Input: part model. Units: mm. Frame: model coordinates. Coordinates: 2 decimals unless noted, no trailing zeros. Write each loop counter-clockwise with the first axis right and the second up, starting at its lowest first coordinate (ties: lowest second). Pieces come first, ordered by that corner, then holes. Notation, with made-up numbers: (19.25, 47.5) - (50.25, 47.5) arc R11 cw to (50.25, 56.5) - close; hole circle Ø11 at (20, 75.25). An arc over 180 degrees is marked (long way). Put each result on its own line as item: value. Start each with the question number.
1. Cut plane B-B, the plane x = 85. Return loops of the section in (y, z).
2. Cut plane D-D, the plane y = 34. Return loops of the section in (x, z), and give its area (3 significant figures).
3. Cut plane C-C, the plane z = 1.15. Return loops of the section in (x, y), and give its area (3 significant figures).
4. Line query: line 1 (Y direction, x = 15, z = 1.2); line 2 (X direction, y = 5.5, z = 1.2); line 3 (X direction, y = 25.5, z = 0.5). Output: solid intervals per line, ascending.
5. Pull-direction query (Y, two-part tool) for faces 1 (the flat face through (49, 26, 0)), 2 (the cylindrical face through (13.4, 46.07, 0.79)); classes: released by +Y, released by -Y, zero draft, split by the parting line, or undercut.
6. Cut plane A-A, the plane y = 46. Return loops of the section in (x, z).
from build123d import *

# Parameters (mm, degrees)
ESQUISSE1_W             = 100
ESQUISSE1_H             = 52
ESQUISSE1_R             = 1.6
BOSS_EXTRU_1_DEPTH      = 1.6
ESQUISSE2_R             = 10
ENL_V_MAT_EXTRU_1_DEPTH = 113.723378232


with BuildPart() as part:
    # Esquisse1 → Boss.-Extru.1 (new body)
    with BuildSketch(Plane.XY):
        with Locations((50, 26)):
            Rectangle(ESQUISSE1_W, ESQUISSE1_H)
        with Locations((15, 46)):
            Circle(ESQUISSE1_R, mode=Mode.SUBTRACT)
        with Locations((85, 46)):
            Circle(ESQUISSE1_R, mode=Mode.SUBTRACT)
        with Locations((15, 6)):
            Circle(ESQUISSE1_R, mode=Mode.SUBTRACT)
        with Locations((85, 6)):
            Circle(ESQUISSE1_R, mode=Mode.SUBTRACT)
    extrude(amount=BOSS_EXTRU_1_DEPTH)

    # Esquisse2 → Enlèv. mat.-Extru.1 (cut, through all)
    with BuildSketch(Plane(origin=(0, 0, 0), x_dir=(-1, 0, 0), z_dir=(0, 0, -1))):
        with Locations((-100, 26)):
            Circle(ESQUISSE2_R)
        with Locations((0, 26)):
            Circle(ESQUISSE2_R)
    extrude(amount=-ENL_V_MAT_EXTRU_1_DEPTH, mode=Mode.SUBTRACT)


solid = part.part
Report:
1. outline: (0, 0) - (4.4, 0) - (4.4, 1.6) - (0, 1.6) - close; (7.6, 0) - (44.4, 0) - (44.4, 1.6) - (7.6, 1.6) - close; (47.6, 0) - (52, 0) - (52, 1.6) - (47.6, 1.6) - close
2. outline: (6, 0) - (94, 0) - (94, 1.6) - (6, 1.6) - close
2. area: 141 mm^2
3. outline: (0, 0) - (100, 0) - (100, 16) arc R10 cw to (100, 36) - (100, 52) - (0, 52) - (0, 36) arc R10 cw to (0, 16) - close; hole circle Ø3.2 at (15, 6); hole circle Ø3.2 at (15, 46); hole circle Ø3.2 at (85, 6); hole circle Ø3.2 at (85, 46)
3. area: 4,850 mm^2
4. line 1: y = 0 to 4.4, 7.6 to 44.4, 47.6 to 52
4. line 2: x = 0 to 13.48, 16.52 to 83.48, 86.52 to 100
4. line 3: x = 9.99 to 90.01
5. face 1: zero draft
5. face 2: undercut
6. outline: (0, 0) - (13.4, 0) - (13.4, 1.6) - (0, 1.6) - close; (16.6, 0) - (83.4, 0) - (83.4, 1.6) - (16.6, 1.6) - close; (86.6, 0) - (100, 0) - (100, 1.6) - (86.6, 1.6) - close
